from build123d import *

# Parameters (mm, degrees)
BOSS_EXTRUDE2_DEPTH      = 1.5
BOSS_EXTRUDE2_DEPTH_BACK = 1.5
SKETCH2_R                = 2
BOSS_EXTRUDE3_DEPTH      = 48
BOSS_EXTRUDE4_DEPTH      = 0.5
BOSS_EXTRUDE4_DEPTH_BACK = 3.5
CUT_EXTRUDE1_DEPTH       = 3
CUT_EXTRUDE2_DEPTH       = 26.3039
FILLET1_R                = 1
CUT_EXTRUDE4_REACH       = 74.305
CUT_EXTRUDE5_REACH       = 43.195
SKETCH10_W               = 3
SKETCH10_H               = 0.141883177


with BuildPart() as part:
    # Sketch1 → Boss-Extrude2 (new, two sides: drawn at the far end of the back side and taken through both)
    with BuildSketch(Plane(origin=(0, 108.422012546, -620.347507802), x_dir=(0, 0, -1), z_dir=(1, 0, 0)).offset(-BOSS_EXTRUDE2_DEPTH_BACK)):
        Polygon((-620.347507802, -60.422012546), (-620.347507802, -108.422012546), (-612.347507802, -108.422012546), (-612.347507802, -103.422012546), (-618.347507802, -103.422012546), (-618.347507802, -67.422012546), (-616.347507802, -67.422012546), (-616.347507802, -93.422012546), (-612.347507802, -93.422012546), (-612.347507802, -64.422012546), (-612.347507802, -60.422012546), align=None)
    extrude(amount=BOSS_EXTRUDE2_DEPTH + BOSS_EXTRUDE2_DEPTH_BACK)

    # Sketch2 → Boss-Extrude3 (add)
    with BuildSketch(Plane(origin=(0, 48, 0), x_dir=(1, 0, 0), z_dir=(0, 1, 0))):
        Circle(SKETCH2_R)
    extrude(amount=-BOSS_EXTRUDE3_DEPTH)

    # Sketch4 → Boss-Extrude4 (add, two sides: drawn at the far end of the back side and taken through both)
    with BuildSketch(Plane.ZY.offset(1.5).offset(-BOSS_EXTRUDE4_DEPTH_BACK)):
        with BuildLine():
            Line((-8, 0), (2, 0))
            ThreePointArc((2, 0), (2.585786438, -1.414213562), (4, -2))
            Line((4, -2), (9, -2))
            ThreePointArc((9, -2), (11.121320344, -2.878679656), (12, -5))
            Line((12, -5), (12, -19))
            ThreePointArc((12, -19), (11.121320344, -21.121320344), (9, -22))
            Line((9, -22), (-15, -22))
            ThreePointArc((-15, -22), (-17.121320344, -21.121320344), (-18, -19))
            Line((-18, -19), (-18, -5))
            ThreePointArc((-18, -5), (-17.121320344, -2.878679656), (-15, -2))
            Line((-15, -2), (-10, -2))
            ThreePointArc((-10, -2), (-8.585786438, -1.414213562), (-8, 0))
        make_face()
        with BuildLine():
            Line((-7, -15), (1, -15))
            ThreePointArc((1, -15), (3, -17), (1, -19))
            Line((1, -19), (-7, -19))
            ThreePointArc((-7, -19), (-9, -17), (-7, -15))
        make_face(mode=Mode.SUBTRACT)
    extrude(amount=BOSS_EXTRUDE4_DEPTH + BOSS_EXTRUDE4_DEPTH_BACK)

    # Sketch6 → Cut-Extrude1 (cut)
    with BuildSketch(Plane.ZY.offset(1.5)):
        Polygon((-6.6312, 18.3509), (-6.6312, 16.6491), (-8.2803, 15), (-10.2803, 15), (-10.2803, 41.5842), (-8.2803, 41.5842), (-6.047, 39.3509), (-6.047, 37.6491), (-6.3619, 37.3342), (-4.8786, 35.8509), (-4.8786, 34.1491), (-6.654, 32.3737), (-6.6312, 32.3509), (-6.6312, 30.6491), (-6.654, 30.6263), (-4.8786, 28.8509), (-4.8786, 27.1491), (-6.0698, 25.9579), (-5.4628, 25.3509), (-5.4628, 23.6491), (-6.654, 22.4579), (-6.047, 21.8509), (-6.047, 20.1491), (-7.2382, 18.9579), align=None)
    extrude(amount=-CUT_EXTRUDE1_DEPTH, mode=Mode.SUBTRACT)

    # Sketch7 → Cut-Extrude2 (cut)
    with BuildSketch(Plane.XZ.offset(-15)):
        Polygon((0, -6.6312), (-1.5, -5.1312), (-1.5, -8), (0, -8), align=None)
    extrude(amount=-CUT_EXTRUDE2_DEPTH, mode=Mode.SUBTRACT)

    # Fillet1
    fillet1_edges = [part.edges().sort_by_distance(p)[0] for p in [
        (0, 41.3039, -7.3156),
    ]]
    fillet(fillet1_edges, radius=FILLET1_R)

    # Cut-Extrude4: up to this plane
    cut_extrude4_end = Plane(origin=(28.627440951, 39.3509, -6.047), z_dir=(2.4829835882571804e-15, 0.7071067811865529, 0.7071067811865422))
    # Sketch9 → Cut-Extrude4 (cut, up to the surface)
    with BuildSketch(Plane(origin=(0, 48, 0), x_dir=(1, 0, 0), z_dir=(0, 1, 0)), mode=Mode.PRIVATE) as cut_extrude4_sk1:
        with BuildLine():
            ThreePointArc((-1.5, 6.5), (-1.060660172, 7.560660172), (0, 8))
            Line((0, 8), (-1.5, 8))
            Line((-1.5, 8), (-1.5, 6.5))
        make_face()
    cut_extrude4_tool1 = split(extrude(cut_extrude4_sk1.sketch, amount=-CUT_EXTRUDE4_REACH, mode=Mode.PRIVATE), bisect_by=cut_extrude4_end, keep=Keep.BOTH, mode=Mode.PRIVATE)
    add(cut_extrude4_tool1.solids().sort_by_distance((-1.164948, 48, -7.664948))[0], mode=Mode.SUBTRACT)
    # Sketch9 → Cut-Extrude4 (cut, up to the surface)
    with BuildSketch(Plane(origin=(0, 48, 0), x_dir=(1, 0, 0), z_dir=(0, 1, 0)), mode=Mode.PRIVATE) as cut_extrude4_sk2:
        with BuildLine():
            Line((1.5, 6.5), (1.5, 8))
            Line((1.5, 8), (0, 8))
            ThreePointArc((0, 8), (1.060660172, 7.560660172), (1.5, 6.5))
        make_face()
    cut_extrude4_tool2 = split(extrude(cut_extrude4_sk2.sketch, amount=-CUT_EXTRUDE4_REACH, mode=Mode.PRIVATE), bisect_by=cut_extrude4_end, keep=Keep.BOTH, mode=Mode.PRIVATE)
    add(cut_extrude4_tool2.solids().sort_by_distance((1.164948, 48, -7.664948))[0], mode=Mode.SUBTRACT)

    # Cut-Extrude5: up to this plane
    cut_extrude5_end = Plane(origin=(28.627440951, 16.6491, -6.6312), z_dir=(2.462807656596698e-15, -0.707106781186546, 0.707106781186549))
    # Sketch10 → Cut-Extrude5 (cut, up to the surface)
    with BuildSketch(Plane(origin=(0, 15, 0), x_dir=(1, 0, 0), z_dir=(0, 1, 0)), mode=Mode.PRIVATE) as cut_extrude5_sk1:
        with Locations((0, 7.929058411)):
            Rectangle(SKETCH10_W, SKETCH10_H)
    cut_extrude5_tool1 = split(extrude(cut_extrude5_sk1.sketch, amount=CUT_EXTRUDE5_REACH, mode=Mode.PRIVATE), bisect_by=cut_extrude5_end, keep=Keep.BOTH, mode=Mode.PRIVATE)
    add(cut_extrude5_tool1.solids().sort_by_distance((0, 15, -7.929058))[0], mode=Mode.SUBTRACT)


solid = part.part
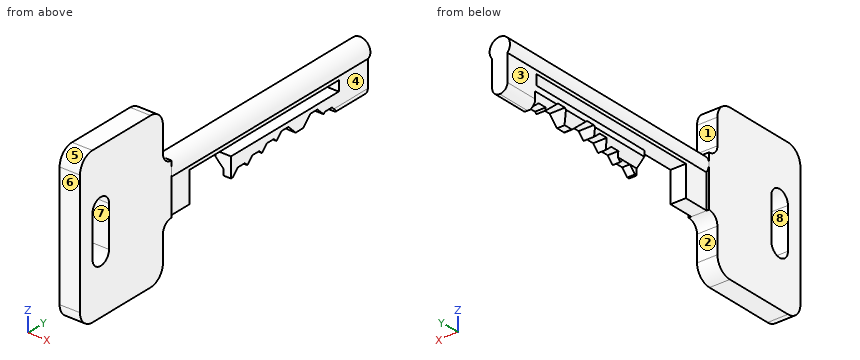
Can you work these out from the model? Positions are in its coordinate system, mm. Face numbers are marked on the shaded views. A direction names the side the tool comes from. Coordinates: 2 decimals unless noted, no trailing zeros. Order: outer loops, then holes, each group sorted by start corner. A loop starts at its lowest first (then second) coordinate and runs counter-clockwise, first axis right, second up. Notation, with made-up numbers: M 25.5,13.5 L 35.5,13.5 A3 ccw 35.5,18.5 Z; hole C -28.75,47.25 d6. An arc over 180 degrees is marked long. Write item = value, one per line.
(1) For the marked faces 1, 2, 3 and 4, which set-ups out of +Z, -Z, +X, -X, +Y, -Y let a thin tool reach every point of the face, with its end or its side?
Results are:
face_1 = +Z, +X, -X, +Y
face_2 = -Z, +X, -X, +Y
face_3 = -Z, -X, +Y
face_4 = -Z, +X, +Y
(2) I need wall thicknesses on line 1 along Y through (x, z) = (-0.7, -2.5); line 2 along Y through (x, z) = (-1.3, -1); line 3 along Y through (x, z) = (0.5, 7.5). Which ranges of each line are inside material? Lowest first, please. Write a range as [from, to].
Results are:
line_1 = [-22, -19], [-15, 5], [41, 48]
line_2 = [-22, -19], [-15, 48]
line_3 = [-22, -2]
(3) Suppose I cut it at C-C on z = 6.25. Please give me the cut outline in (x, y).
Results are:
outline = M -2,-22 L 2,-22 L 2,-2 L -2,-2 Z
(4) For pin 1 Ø5.5 at (y, z) = (21, -3.5) entering from +X; pin 2 Ø1.6 at (x, y) = (1, 17.5) entering from -Z; pin 3 Ø1 at (y, z) = (16, -7.5) entering from -X, each with a flat end and sliding along its axis, tell me the tip position at first contact or that it passes through.
Results are:
pin_1 = 1.85
pin_2 = -6.63
pin_3 = 0
(5) Suppose I cut it at A-A on z = -2.75. Please give me the cut outline in (x, y).
Results are:
outline = M -2,-22 L 2,-22 L 2,-19 L -2,-19 Z; M -2,-15 L 2,-15 L 2,0 L 1.5,0 L 1.5,5 L -1.5,5 L -1.5,0 L -2,0 Z; M -1.5,41 L 1.5,41 L 1.5,48 L -1.5,48 Z
(6) Suppose I cut it at B-B on y = 7. Please give me the cut outline in (x, z).
Results are:
outline = M -1.5,-2 L 1.5,-2 L 1.5,-1.32 A2 ccw long -1.5,-1.32 Z
(7) If we mould it in two halves opening along Z, with no side actions, what happens to the marked faces 5, 6, 7 and 8? For each: pulls with the +Z half, pulls with the -Z half, needs draft (parallel to the pull), parting line crosses it, or undercut.
Results are:
face_5 = pulls with the +Z half
face_6 = needs draft
face_7 = undercut
face_8 = undercut
